Work out the finished part from the listing and answer in its coordinate system (mm). Coordinates: 2 decimals unless noted, no trailing zeros. Order: outer loops, then holes, each group sorted by start corner. A loop starts at its lowest first (then second) coordinate and runs counter-clockwise, first axis right, second up. Notation, with made-up numbers: (37, -33) - (56, -33) arc R21 cw to (56, -25) - close; hole circle Ø8 at (40.25, 17.5). An arc over 180 degrees is marked (long way). Answer as a JSON object with one key per item and string values. Group by question number.
1) Section C-C (y = 30) is taken. Give the vertices of the cut face in (x, z).
2) Section A-A (z = 154) is taken. Give the vertices of the cut face in (x, y), plus the area to 3 significant figures.
3) Section D-D (z = 198) is taken. Give the vertices of the cut face in (x, y), plus the area to 3 significant figures.
4) Section B-B (x = -67) is taken. Give the vertices of the cut face in (y, z), plus the area to 3 significant figures.
5) Find the intervals of material crossed by line 1 along Z through (x, y) = (75, 7); line 2 along X through (y, z) = (40, 170); line 3 along Y through (x, z) = (37.5, 192), in increasing order.
6) Each of these flat-tipped pins is pushed along its axis until it touches: P1, Ø6, axis at x = -82.5, y = 42.5, coming from the -Z side; P2, Ø1.4, axis at y = 2.5, z = 197.5, coming from the +X side; P3, Ø3, axis at y = 7, z = 199.5, coming from the -X side. Where does it stop, or does it pass through?
from build123d import *

# Parameters (mm, degrees)
ESQUISSE1_R             = 3
BOSS_EXTRU_1_DEPTH      = 200
ESQUISSE4_W             = 5
ESQUISSE4_H             = 50
BOSS_EXTRU_4_DEPTH      = 180
BOSS_EXTRU_7_DEPTH      = 50
ESQUISSE6_W             = 20
ESQUISSE6_H             = 10.719834163
ENL_V_MAT_EXTRU_2_DEPTH = 10
ESQUISSE5_W             = 10
ESQUISSE5_H             = 10
ENL_V_MAT_EXTRU_1_DEPTH = 10
ESQUISSE14_R            = 5
ENL_V_MAT_EXTRU_4_DEPTH = 15
BOSS_EXTRU_8_REACH      = 242.401
ENL_V_MAT_EXTRU_5_REACH = 238.046
ESQUISSE16_W            = 190
ESQUISSE16_H            = 150


with BuildPart() as part:
    # Esquisse1 → Boss.-Extru.1 (new body)
    with BuildSketch(Plane.XY):
        Polygon((-105.796013405, 0), (84.203986595, 0), (84.203986595, 33.502126335), (-105.796013405, 2), align=None)
        with Locations((69.406004871, 22.939397164)):
            Circle(ESQUISSE1_R, mode=Mode.SUBTRACT)
        with Locations((40.981469067, 6.77616521)):
            Circle(ESQUISSE1_R, mode=Mode.SUBTRACT)
        with Locations((-40.796013405, 6)):
            Circle(ESQUISSE1_R, mode=Mode.SUBTRACT)
        with Locations((8.861542866, 12.901085106)):
            Circle(ESQUISSE1_R, mode=Mode.SUBTRACT)
    extrude(amount=BOSS_EXTRU_1_DEPTH)

    # Esquisse4 → Boss.-Extru.4 (add)
    with BuildSketch(Plane(origin=(84.203986595, 0, 0), x_dir=(0, 0, -1), z_dir=(1, 0, 0))):
        with Locations((-202.5, 25)):
            Rectangle(ESQUISSE4_W, ESQUISSE4_H)
        with Locations((2.5, 25)):
            Rectangle(ESQUISSE4_W, ESQUISSE4_H)
    extrude(amount=-BOSS_EXTRU_4_DEPTH)

    # Esquisse8 → Boss.-Extru.7 (add)
    with BuildSketch(Plane(origin=(0, 50, 0), x_dir=(1, 0, 0), z_dir=(0, 1, 0))):
        Polygon((84.203986595, 0), (-95.796013405, 0), (-95.796013405, -5), align=None)
    boss_extru_7 = extrude(amount=-BOSS_EXTRU_7_DEPTH)

    # Esquisse6 → Enlèv. mat.-Extru.2 (cut)
    with BuildSketch(Plane(origin=(0, 0, -5), x_dir=(-1, 0, 0), z_dir=(0, 0, -1))):
        with Locations((95.796013405, 5.359917081)):
            Rectangle(ESQUISSE6_W, ESQUISSE6_H)
    enl_v_mat_extru_2 = extrude(amount=-ENL_V_MAT_EXTRU_2_DEPTH, mode=Mode.SUBTRACT)

    # Esquisse5 → Enlèv. mat.-Extru.1 (cut)
    with BuildSketch(Plane(origin=(84.203986595, 0, 0), x_dir=(0, 0, -1), z_dir=(1, 0, 0))):
        with Locations((-200, 5)):
            Rectangle(ESQUISSE5_W, ESQUISSE5_H)
        with Locations((0, 5)):
            Rectangle(ESQUISSE5_W, ESQUISSE5_H)
    extrude(amount=-ENL_V_MAT_EXTRU_1_DEPTH, mode=Mode.SUBTRACT)

    # Esquisse14 → Enlèv. mat.-Extru.4 (cut)
    with BuildSketch(Plane(origin=(0, 0, -5), x_dir=(-1, 0, 0), z_dir=(0, 0, -1))):
        with Locations((-69.406004871, 22.939397164)):
            Circle(ESQUISSE14_R)
        with Locations((-40.981469067, 6.77616521)):
            Circle(ESQUISSE14_R)
        with Locations((-8.861542866, 12.901085106)):
            Circle(ESQUISSE14_R)
        with Locations((40.796013405, 6)):
            Circle(ESQUISSE14_R)
    enl_v_mat_extru_4 = extrude(amount=-ENL_V_MAT_EXTRU_4_DEPTH, mode=Mode.SUBTRACT)

    # Symétrie3: Boss.-Extru.7, Enlèv. mat.-Extru.2, Enlèv. mat.-Extru.4 across plane
    add(boss_extru_7.mirror(Plane(origin=(0, 0, 100), x_dir=(1, 0, 0), z_dir=(0, 0, -1))))
    add(enl_v_mat_extru_2.mirror(Plane(origin=(0, 0, 100), x_dir=(1, 0, 0), z_dir=(0, 0, -1))), mode=Mode.SUBTRACT)
    add(enl_v_mat_extru_4.mirror(Plane(origin=(0, 0, 100), x_dir=(1, 0, 0), z_dir=(0, 0, -1))), mode=Mode.SUBTRACT)

    # Boss.-Extru.8: up to this plane
    boss_extru_8_end = Plane(origin=(-95.796013405, -180.069431054, 195), z_dir=(-0.0277670672403533, 0, 0.9996144206527183))
    # Esquisse15 → Boss.-Extru.8 (add, up to the surface)
    with BuildSketch(Plane(origin=(0, 0, -5), x_dir=(-1, 0, 0), z_dir=(0, 0, -1)), mode=Mode.PRIVATE) as boss_extru_8_sk1:
        Polygon((-84.203986595, 33.502126335), (-79.203986595, 32.67312301), (-79.203986595, 50), (-84.203986595, 50), align=None)
    boss_extru_8_tool1 = split(extrude(boss_extru_8_sk1.sketch, amount=-BOSS_EXTRU_8_REACH, mode=Mode.PRIVATE), bisect_by=boss_extru_8_end, keep=Keep.BOTH, mode=Mode.PRIVATE)
    add(boss_extru_8_tool1.solids().sort_by_distance((81.683563, 41.542119, -5))[0])

    # Enlèv. mat.-Extru.5: up to this face of the body (flat: up to its plane)
    enl_v_mat_extru_5_end = Plane(part.part.faces().sort_by_distance((-10.38578146, 0, 100.003530671))[0])
    # Esquisse16 → Enlèv. mat.-Extru.5 (cut, up to the picked face)
    with BuildSketch(Plane(origin=(0, 50, 0), x_dir=(1, 0, 0), z_dir=(0, 1, 0)), mode=Mode.PRIVATE) as enl_v_mat_extru_5_sk1:
        with Locations((-10.796013405, -70)):
            Rectangle(ESQUISSE16_W, ESQUISSE16_H)
    enl_v_mat_extru_5_tool1 = split(extrude(enl_v_mat_extru_5_sk1.sketch, amount=-ENL_V_MAT_EXTRU_5_REACH, mode=Mode.PRIVATE), bisect_by=enl_v_mat_extru_5_end, keep=Keep.BOTH, mode=Mode.PRIVATE)
    add(enl_v_mat_extru_5_tool1.solids().sort_by(Axis((-10.796013, 50, 70), (0, -1, 0)))[0], mode=Mode.SUBTRACT)


solid = part.part
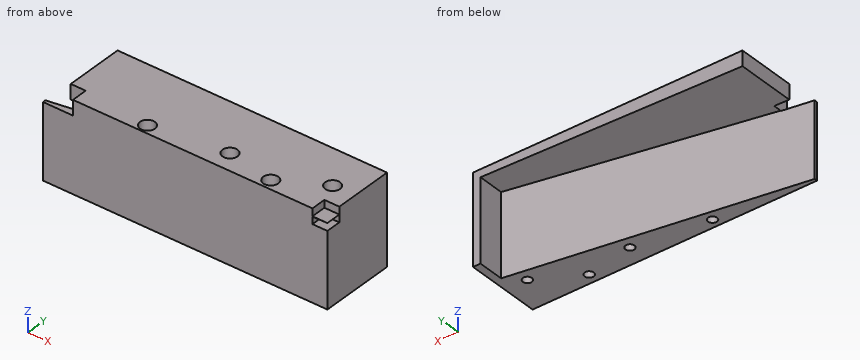
Report:
{
 "1": {"outline": "(-95.8, 195) - (63.08, 199.41) - (63.08, 145) - (84.2, 145) - (84.2, 205) - (-95.8, 205) - close"},
 "2": {"outline": "(-105.8, 0) - (84.2, 0) - (84.2, 50) - (79.2, 50) - (79.2, 32.67) - (-105.8, 2) - close; hole circle Ø6 at (-40.8, 6); hole circle Ø6 at (8.86, 12.9); hole circle Ø6 at (40.98, 6.78); hole circle Ø6 at (69.41, 22.94)", "area": "3,340 mm²"},
 "3": {"outline": "(-95.8, 10.72) - (-85.8, 10.72) - (-85.8, 0) - (74.2, 0) - (74.2, 10) - (84.2, 10) - (84.2, 50) - (79.2, 50) - (79.2, 32.67) - (12.2, 21.56) - (12.2, 50) - (-95.8, 50) - close; hole circle Ø10 at (-40.8, 6); hole circle Ø10 at (8.86, 12.9); hole circle Ø10 at (40.98, 6.78); hole circle Ø10 at (69.41, 22.94)", "area": "6,950 mm²"},
 "4": {"outline": "(0, 145) - (8.43, 145) - (8.43, 195.8) - (50, 195.8) - (50, 205) - (0, 205) - close", "area": "888 mm²"},
 "5": {"line 1": "z = 145 to 195, 199.74 to 200", "line 2": "x = 79.2 to 84.2", "line 3": "y = 0 to 3.19, 10.36 to 25.76"},
 "6": {"P1": "stops at z = 195.29", "P2": "stops at x = 74.2", "P3": "stops at x = -85.8"}
}
